The model under review builds one solid part; all positions refer to its coordinate system, in mm. Face numbers are marked on the shaded views. A direction names the side the tool comes from. Round coordinates to 2 decimals unless told otherwise and drop trailing zeros. Order: outer loops, then holes, each group sorted by start corner. A loop starts at its lowest first (then second) coordinate and runs counter-clockwise, first axis right, second up. Notation, with made-up numbers: (-0.75, 84.5) -> (38.25, 84.5) arc R26 ccw to (38.25, 107.5) -> close; hole circle Ø4 at (50.25, -12.5). An arc over 180 degrees is marked (long way). Use a Markdown table: item, result. Add a question column.
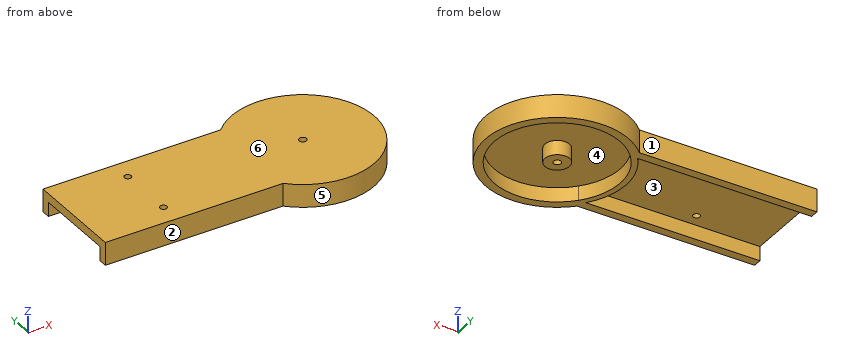
```python
from build123d import *

# Parameters (mm, degrees)
DODANIE_WYCI_GNI_CIE1_DEPTH = 8
OTW_R_POD_RUB_M22_D         = 2.6
SKORUPA1_T                  = -3
DODANIE_WYCI_GNI_CIE2_REACH = 228.526
OTW_R_POD_RUB_M21_D         = 2.6
WYTNIJ_WYCI_GNI_CIE1_REACH  = 228.526
SZKIC7_W                    = 41
SZKIC7_H                    = 21
OTWORY_USTALAJ_CE_8_0MM1_D  = 8
SZKIC18_W                   = 8
SZKIC18_H                   = 6
SZKIC18_W_2                 = 6
SZKIC18_H_2                 = 4
DODANIE_WYCI_GNI_CIE3_DEPTH = 10
SZYK_LINIOWY1_COUNT         = 2
SZYK_LINIOWY1_PITCH         = 50
OTW_R_POD_RUB_M24_D         = 2.4


with BuildPart() as part:
    # Szkic1 → Dodanie-wyciągnięcie1 (new body)
    with BuildSketch(Plane.XY):
        with BuildLine():
            Line((17.853571071, 17.5), (182.146428929, 17.5))
            ThreePointArc((182.146428929, 17.5), (225, 0), (182.146428929, -17.5))
            Line((182.146428929, -17.5), (17.853571071, -17.5))
            ThreePointArc((17.853571071, -17.5), (-25, 0), (17.853571071, 17.5))
        make_face()
    extrude(amount=DODANIE_WYCI_GNI_CIE1_DEPTH)

    # Otwór pod śrubę M22 (through all)
    with Locations(Plane(origin=(0, 0, 8), x_dir=(-1, 0, 0), z_dir=(0, 0, 1))):
        with Locations((-200, 0)):
            Hole(OTW_R_POD_RUB_M22_D / 2)

    # Skorupa1
    skorupa1_openings = [part.faces().sort_by_distance(p)[0] for p in [
        (99.943079522, 0, 0),
    ]]
    offset(amount=SKORUPA1_T, openings=skorupa1_openings, kind=Kind.INTERSECTION)

    # Szkic15 → Dodanie-wyciągnięcie2 (add, up to next)
    with BuildSketch(Plane(origin=(0, 0, 0), x_dir=(-1, 0, 0), z_dir=(0, 0, -1)), mode=Mode.PRIVATE) as dodanie_wyci_gni_cie2_sk1:
        with BuildLine():
            Line((-16.545392108, -14.5), (-19.124591499, -14.5))
            ThreePointArc((-19.124591499, -14.5), (-24, 0), (-19.124591499, 14.5))
            Line((-19.124591499, 14.5), (-16.545392108, 14.5))
            ThreePointArc((-16.545392108, 14.5), (-22, 0), (-16.545392108, -14.5))
        make_face()
    dodanie_wyci_gni_cie2_tool1 = extrude(dodanie_wyci_gni_cie2_sk1.sketch, amount=-DODANIE_WYCI_GNI_CIE2_REACH, mode=Mode.PRIVATE) - part.part
    # Szkic15 → Dodanie-wyciągnięcie2 (add, up to next)
    with BuildSketch(Plane(origin=(0, 0, 0), x_dir=(-1, 0, 0), z_dir=(0, 0, -1)), mode=Mode.PRIVATE) as dodanie_wyci_gni_cie2_sk2:
        with BuildLine():
            Line((-180.875408501, -14.5), (-183.454607892, -14.5))
            ThreePointArc((-183.454607892, -14.5), (-178, 0), (-183.454607892, 14.5))
            Line((-183.454607892, 14.5), (-180.875408501, 14.5))
            ThreePointArc((-180.875408501, 14.5), (-176, 0), (-180.875408501, -14.5))
        make_face()
    dodanie_wyci_gni_cie2_tool2 = extrude(dodanie_wyci_gni_cie2_sk2.sketch, amount=-DODANIE_WYCI_GNI_CIE2_REACH, mode=Mode.PRIVATE) - part.part
    add(dodanie_wyci_gni_cie2_tool1.solids().sort_by_distance((17.834992, 14.200572, 0))[0])
    add(dodanie_wyci_gni_cie2_tool2.solids().sort_by_distance((182.165008, -14.200572, 0))[0])

    # Otwór pod śrubę M21 (through all)
    with Locations(Plane.XY.offset(8)):
        with Locations((7.1, 0), (-7.1, 0)):
            Hole(OTW_R_POD_RUB_M21_D / 2)

    # Szkic7 → Wytnij-wyciągnięcie1 (cut, up to next)
    with BuildSketch(Plane(origin=(0, 0, 0), x_dir=(-1, 0, 0), z_dir=(0, 0, -1)), mode=Mode.PRIVATE) as wytnij_wyci_gni_cie1_sk1:
        with Locations((-55, 0)):
            Rectangle(SZKIC7_W, SZKIC7_H)
    wytnij_wyci_gni_cie1_tool1 = extrude(wytnij_wyci_gni_cie1_sk1.sketch, amount=-WYTNIJ_WYCI_GNI_CIE1_REACH, mode=Mode.PRIVATE) & part.part
    add(wytnij_wyci_gni_cie1_tool1.solids().sort_by_distance((55, 0, 0))[0], mode=Mode.SUBTRACT)

    # Otwory ustalające Ø8.0mm1 (through all)
    with Locations(Plane(origin=(0, 0, 8), x_dir=(-1, 0, 0), z_dir=(0, 0, 1))):
        with Locations((0, 0)):
            Hole(OTWORY_USTALAJ_CE_8_0MM1_D / 2)

    # Szkic18 → Dodanie-wyciągnięcie3 (add)
    with BuildSketch(Plane(origin=(50, 0, 0), x_dir=(0, 0, -1), z_dir=(1, 0, 0))):
        with Locations((-4, 20.5)):
            Rectangle(SZKIC18_W, SZKIC18_H)
        with Locations((-4, 20.5)):
            Rectangle(SZKIC18_W_2, SZKIC18_H_2, mode=Mode.SUBTRACT)
    dodanie_wyci_gni_cie3 = extrude(amount=DODANIE_WYCI_GNI_CIE3_DEPTH)

    # Szyk liniowy1: Dodanie-wyciągnięcie3 ×2
    with Locations(*[(i * SZYK_LINIOWY1_PITCH, 0, 0) for i in range(1, SZYK_LINIOWY1_COUNT)]):
        add(dodanie_wyci_gni_cie3)

    # Otwór pod śrubę M24 (through all)
    with Locations(Plane(origin=(0, 0, 5), x_dir=(-1, 0, 0), z_dir=(0, 0, -1))):
        with Locations((-145, -10), (-145, 10), (-95, 10), (-95, -10)):
            Hole(OTW_R_POD_RUB_M24_D / 2)

    # Cięcie powierzchnią1
    split(bisect_by=Plane(origin=(120, 0, 0), x_dir=(0, 0, -1), z_dir=(1, 0, 0)), keep=Keep.TOP)


solid = part.part
```
Q1. To check wall thickness, follow line 1 along Y through (x, z) = (145, 6.3); line 2 along Y through (x, z) = (200, 2); line 3 along Y through (x, z) = (129, 2.5). State the ranges of each line that lie inside material, in increasing order.
Q2. Draft analysis for pull direction X (two halves, no side actions). For the marked faces 4, 5 and 6, state which applies: released by +X, released by -X, zero draft, split by the parting line, or undercut.
Q3. For the marked faces 1, 2 and 3, list the 3-axis set-ups (+Z, -Z, +X, -X, +Y, -Y) from which the entire face can be reached by the end or side of a thin tool; tool diameter is ignored.
Q4. Add section A-A, the plane z = 4. Give the boundary of the cut face in (x, y).
Q5. Add section D-D, the plane y = -15.5. Give the boundary of the cut face in (x, z), then the cut area to 3 significant figures.
Q6. Add section B-B, the plane x = 145. Give the boundary of the cut face in (y, z), then the cut area to 3 significant figures.
Q7. For pin 1 (1.5 mm diameter, centred on x = 144.5, z = 3.5, fed in from +Y); pin 2 (14.5 mm diameter, centred on x = 145.5, y = 1.5, fed in from -Z); pin 3 (1.5 mm diameter, centred on y = -5.5, z = 1.5, fed in from +X); pin 4 (2 mm diameter, centred on x = 145, y = -10, fed in from -Z), all flat-tipped, find the tip position at first contact; note any pin that passes through.
Q8. Add section C-C, the plane y = 10. Give the boundary of the cut face in (x, z).
Return value:
| question | item | result |
|---|---|---|
| 1 | line 1 | -17.5 to -11.2, -8.8 to 8.8, 11.2 to 17.5 |
| 1 | line 2 | -25 to -22, -4.3 to -1.3, 1.3 to 4.3, 22 to 25 |
| 1 | line 3 | -17.5 to -14.5, 14.5 to 17.5 |
| 2 | face 4 | undercut |
| 2 | face 5 | split by the parting line |
| 2 | face 6 | zero draft |
| 3 | face 1 | +Z, -Z, -X, +Y |
| 3 | face 2 | +Z, -Z, -X, -Y |
| 3 | face 3 | -Z, -X |
| 4 | outline | (120, -17.5) -> (182.15, -17.5) arc R25 ccw (long way) to (182.15, 17.5) -> (120, 17.5) -> (120, 14.5) -> (180.88, 14.5) arc R24 ccw to (180.88, -14.5) -> (120, -14.5) -> close; circle Ø8.6 at (200, 0); hole circle Ø44 at (200, 0); hole circle Ø2.6 at (200, 0) |
| 5 | outline | (120, 0) -> (184.39, 0) -> (184.39, 5) -> (215.61, 5) -> (215.61, 0) -> (219.62, 0) -> (219.62, 8) -> (120, 8) -> close |
| 5 | area | 641 mm² |
| 6 | outline | (-17.5, 0) -> (-14.5, 0) -> (-14.5, 5) -> (-11.2, 5) -> (-11.2, 8) -> (-17.5, 8) -> close; (-8.8, 5) -> (8.8, 5) -> (8.8, 8) -> (-8.8, 8) -> close; (11.2, 5) -> (14.5, 5) -> (14.5, 0) -> (17.5, 0) -> (17.5, 8) -> (11.2, 8) -> close |
| 6 | area | 121 mm² |
| 7 | pin 1 | y = 17.5 |
| 7 | pin 2 | z = 5 |
| 7 | pin 3 | x = 224.54 |
| 7 | pin 4 | through |
| 8 | outline | (120, 5) -> (143.8, 5) -> (143.8, 8) -> (120, 8) -> close; (146.2, 5) -> (178.18, 5) -> (178.18, 0) -> (180.4, 0) -> (180.4, 5) -> (219.6, 5) -> (219.6, 0) -> (222.91, 0) -> (222.91, 8) -> (146.2, 8) -> close |
